Verification items for the finished model (mm, model axes). Round coordinates to 2 decimals unless told otherwise and drop trailing zeros. Order: outer loops, then holes, each group sorted by start corner. A loop starts at its lowest first (then second) coordinate and runs counter-clockwise, first axis right, second up. Notation, with made-up numbers: M 3.25,-32 L 37.25,-32 A22 ccw 37.25,-7 Z; hole C 84.25,31.5 d1. An arc over 180 degrees is marked long. Return JSON: item names as keys, results as strings. Group by question number.
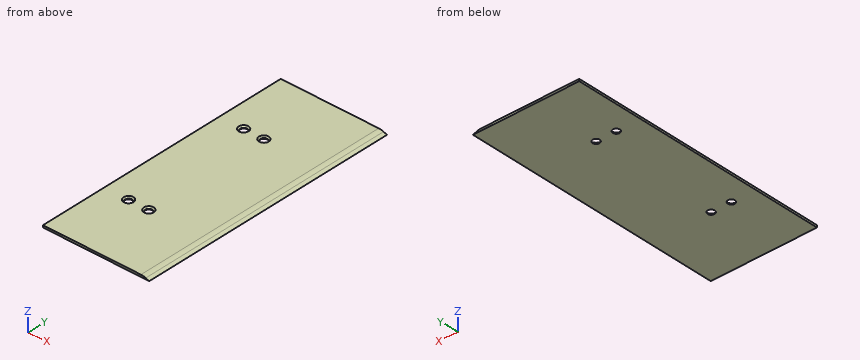
from build123d import *

# Parameters (mm, degrees)
ESQUISSE1_W        = 75.282935443
ESQUISSE1_H        = 186
ESQUISSE1_R        = 2.5
BOSS_EXTRU_1_DEPTH = 1.5
CHANFREIN3_SIZE    = 1.5
CHANFREIN3_SIZE_2  = 4.121216129
CONG_2_R           = 10
CHANFREIN4_SIZE    = 1


with BuildPart() as part:
    # Esquisse1 → Boss.-Extru.1 (new body)
    with BuildSketch(Plane.XY):
        with Locations((10.271299444, 45)):
            Rectangle(ESQUISSE1_W, ESQUISSE1_H)
        with Locations((-10.20705442, 90)):
            Circle(ESQUISSE1_R, mode=Mode.SUBTRACT)
        with Locations((4.153227182, 90)):
            Circle(ESQUISSE1_R, mode=Mode.SUBTRACT)
        with Locations((-10.20705442, 0)):
            Circle(ESQUISSE1_R, mode=Mode.SUBTRACT)
        with Locations((4.153227182, 0)):
            Circle(ESQUISSE1_R, mode=Mode.SUBTRACT)
    extrude(amount=BOSS_EXTRU_1_DEPTH)

    # Chanfrein3
    # the kernel refuses this chamfer: 4.121216129, 1.5 mm, written as the material it takes off along each edge
    with BuildSketch(Plane(origin=(47.912767165, 148.691237174, 1.5), x_dir=(0.09904090225205177, 0, -0.9950833631817484), z_dir=(0, -1, 0))) as chanfrein3_piece_1:
        Polygon((CHANFREIN3_SIZE * 0.995083363182, -CHANFREIN3_SIZE * 0.0990409022521), (-CHANFREIN3_SIZE_2 * 0.0990409022564, -CHANFREIN3_SIZE_2 * 0.995083363226), (0, 0), align=None)
    extrude(amount=207.382474348, mode=Mode.SUBTRACT)

    # Congé2
    cong_2_edges = [part.edges().sort_by_distance(p)[0] for p in [
        (43.791551035, 45, 1.5),
    ]]
    fillet(cong_2_edges, radius=CONG_2_R)

    # Chanfrein4
    chanfrein4_edges = [part.edges().sort_by_distance(p)[0] for p in [
        (-12.70705442, 90, 1.5),
        (1.653227182, 90, 1.5),
        (-12.70705442, 0, 1.5),
        (1.653227182, 0, 1.5),
    ]]
    chamfer(chanfrein4_edges, length=CHANFREIN4_SIZE)


solid = part.part
1. Go/stop test with flat-tipped pins: pin 1 (4 mm diameter, centred on x = -10.21, y = 0, fed in from +Z); pin 2 (6 mm diameter, centred on x = 4.15, y = 90, fed in from +Z). Record where each tip stops, or that it passes through.
2. Cross-section at A-A (y = 0). Enter the section's corners in (x, z).
3. Thickness scan on line 1 along Y through (x, z) = (-11, 0.45); line 2 along Y through (x, z) = (5.5, 0.55); line 3 along Z through (x, y) = (43.5, 29). Record the ranges inside material, lowest first. Write a range as from..to.
4. Cross-section at B-B (y = 96). Enter the section's corners in (x, z), plus the area to 3 significant figures.
Computed:
{
 "1": {"pin 1": "passes through", "pin 2": "stops at z = 1"},
 "2": {"outline": "M -27.37,0 L -12.71,0 L -12.71,0.5 L -13.71,1.5 L -27.37,1.5 Z; M -7.71,0 L 1.65,0 L 1.65,0.5 L 0.65,1.5 L -6.71,1.5 L -7.71,0.5 Z; M 6.65,0 L 47.91,0 L 45.45,0.9 A10 ccw 42.03,1.5 L 7.65,1.5 L 6.65,0.5 Z"},
 "3": {"line 1": "y = -48..-2.37, 2.37..87.63, 92.37..138", "line 2": "y = -48..-2.17, 2.17..87.83, 92.17..138", "line 3": "z = 0..1.39"},
 "4": {"outline": "M -27.37,0 L 47.91,0 L 45.45,0.9 A10 ccw 42.03,1.5 L -27.37,1.5 Z", "area": "110 mm²"}
}
